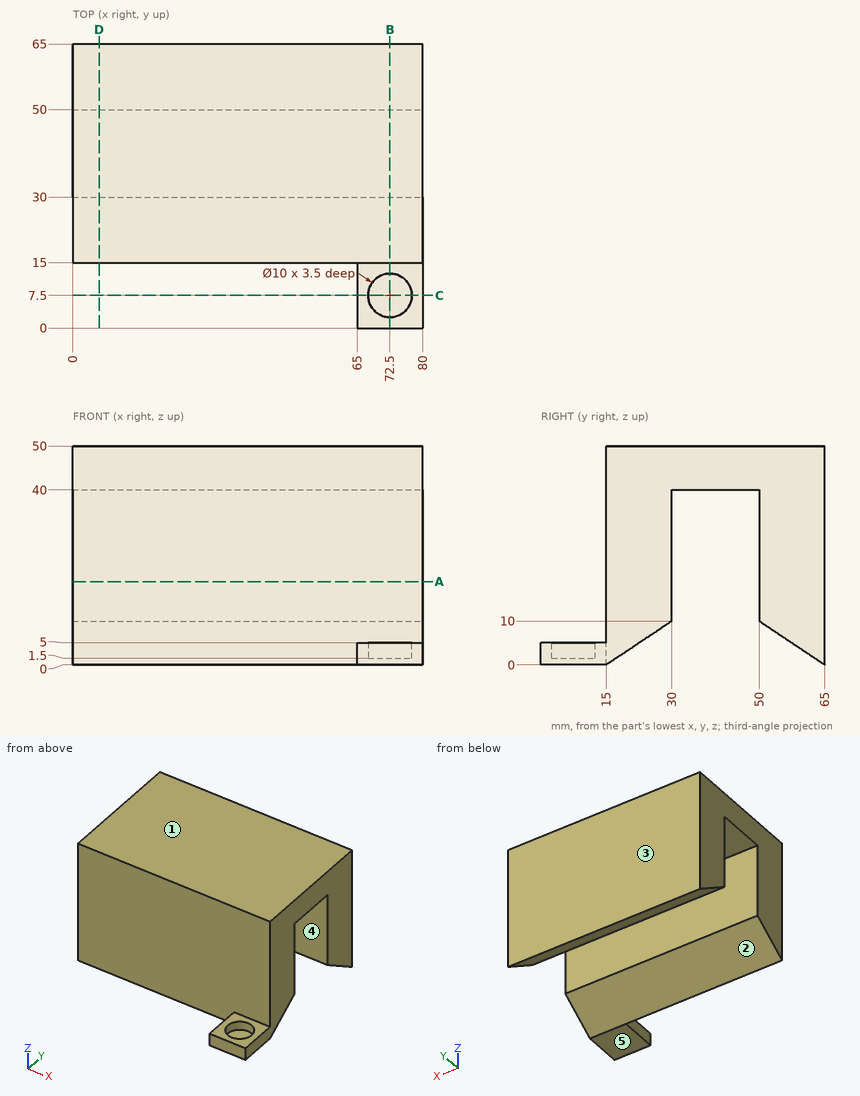
For this review, use the dimensioned drawing (mm, ordinates from the lowest corner) and the shaded views. A direction names the side the tool comes from. Give positions to 0.01 mm unless a question says otherwise; leave off trailing zeros. Write each loop counter-clockwise with the first axis right and the second up, starting at its lowest first coordinate (ties: lowest second). Pieces come first, ordered by that corner, then holes.
(1) Consider section D-D, the plane x = 6. Give the boundary of the cut face in (y, z).
(2) Consider section A-A, the plane z = 19. Give the boundary of the cut face in (x, y), and give its area (3 significant figures).
(3) For P1, Ø24, axis at x = 58, z = 29.5, coming from the -Y side; P2, Ø4, axis at y = 46.5, z = 29, coming from the -X side; P3, Ø3, axis at x = 32, y = 22.5, coming from the -Z side; P4, Ø12, axis at x = 25, y = 56.5, coming from the -Z side, all flat-tipped, find the tip position at first contact; note any pin that passes through.
(4) Tool access review of the marked faces 1 and 2: name each direction out of +Z, -Z, +X, -X, +Y, -Y from which nothing blocks a thin tool from reaching the whole face with its end or side.
(5) Consider section C-C, the plane y = 7.5. Give the boundary of the cut face in (x, z).
(6) The part is to be moulded in two halves that separate along Y. For the marked faces 3, 4 and 5, say which applies: released by +Y, released by -Y, zero draft, split by the parting line, or undercut.
(7) To check wall thickness, follow L1, parallel to Y at x = 72.5, z = 2.6; L2, parallel to Y at x = 19, z = 10; L3, parallel to Y at x = 72.5, z = 2.4. State the ranges of each line that lie inside material, in increasing order.
(8) Consider section B-B, the plane x = 72.5. Give the boundary of the cut face in (y, z).
Returned:
1. outline: (15, 0) - (30, 10) - (30, 40) - (50, 40) - (50, 10) - (65, 0) - (65, 50) - (15, 50) - close
2. outline: (0, 15) - (80, 15) - (80, 30) - (0, 30) - close; (0, 50) - (80, 50) - (80, 65) - (0, 65) - close
2. area: 2,400 mm2
3. P1: stops at y = 15
3. P2: passes through
3. P3: stops at z = 4
3. P4: stops at z = 1.67
4. face 1: +Z, +X, -X, +Y, -Y
4. face 2: -Z, +X, -X
5. outline: (65, 0) - (80, 0) - (80, 5) - (77.5, 5) - (77.5, 1.5) - (67.5, 1.5) - (67.5, 5) - (65, 5) - close
6. face 3: released by +Y
6. face 4: undercut
6. face 5: zero draft
7. L1: y = 0 to 2.5, 12.5 to 18.9, 61.1 to 65
7. L2: y = 15 to 30, 50 to 65
7. L3: y = 0 to 2.5, 12.5 to 18.6, 61.4 to 65
8. outline: (0, 0) - (15, 0) - (30, 10) - (30, 40) - (50, 40) - (50, 10) - (65, 0) - (65, 50) - (15, 50) - (15, 5) - (12.5, 5) - (12.5, 1.5) - (2.5, 1.5) - (2.5, 5) - (0, 5) - close
